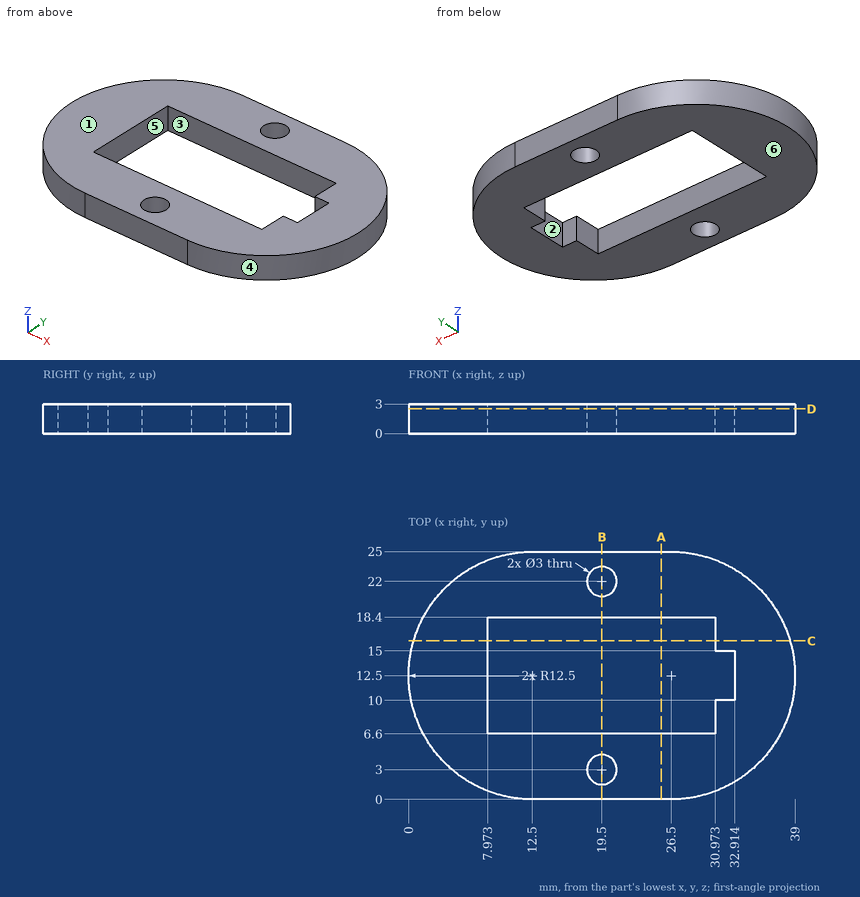
Drawing for the job (mm, zero at the part's lowest x, y, z). A direction names the side the tool comes from. Round coordinates to 2 decimals unless told otherwise and drop trailing zeros. Write each loop counter-clockwise with the first axis right and the second up, starting at its lowest first coordinate (ties: lowest second). Pieces come first, ordered by that corner, then holes. Notation, with made-up numbers: M -17,-38.5 L 1,-38.5 A14 cw 1,-24.5 Z; hole C -33,62 d4. An arc over 180 degrees is marked long. Answer in a Markdown table with one row per item.
1. Saw through at A-A (x = 25.5). List the corners of the cut face in (y, z).
Geometry check:
| item | result |
|---|---|
| outline | M 0,0 L 6.6,0 L 6.6,3 L 0,3 Z; M 18.4,0 L 25,0 L 25,3 L 18.4,3 Z |
2. Saw through at B-B (x = 19.5). List the corners of the cut face in (y, z), and give its area (3 significant figures).
Geometry check:
| item | result |
|---|---|
| outline | M 0,0 L 1.5,0 L 1.5,3 L 0,3 Z; M 4.5,0 L 6.6,0 L 6.6,3 L 4.5,3 Z; M 18.4,0 L 20.5,0 L 20.5,3 L 18.4,3 Z; M 23.5,0 L 25,0 L 25,3 L 23.5,3 Z |
| area | 21.6 mm2 |
3. Saw through at D-D (z = 2.5). List the corners of the cut face in (x, y).
Geometry check:
| item | result |
|---|---|
| outline | M 12.5,0 L 26.5,0 A12.5 ccw 26.5,25 L 12.5,25 A12.5 ccw Z; hole M 7.97,6.6 L 30.97,6.6 L 30.97,10 L 32.91,10 L 32.91,15 L 30.97,15 L 30.97,18.4 L 7.97,18.4 Z; hole C 19.5,3 d3; hole C 19.5,22 d3 |
4. Which spindle directions (+Z, -Z, +X, -X, +Y, -Y) get a long thin tool onto all of the face, cutting with end or side? Do the marked faces 5 and 6. Say none if no direction does.
Geometry check:
| item | result |
|---|---|
| face 5 | +Z, -Z |
| face 6 | -Z, +X, -X, +Y, -Y |
5. Saw through at C-C (y = 16). List the corners of the cut face in (x, z), and give its area (3 significant figures).
Geometry check:
| item | result |
|---|---|
| outline | M 0.5,0 L 7.97,0 L 7.97,3 L 0.5,3 Z; M 30.97,0 L 38.5,0 L 38.5,3 L 30.97,3 Z |
| area | 45.0 mm2 |
6. Probe L1, parallel to Y at x = 19.5, z = 2.3; L2, parallel to Y at x = 25, z = 0.35; L3, parallel to X at y = 12.5, z = 1.45. List the from-to ranges inside material, lowest first. Write a range as [from, to].
Geometry check:
| item | result |
|---|---|
| L1 | [0, 1.5], [4.5, 6.6], [18.4, 20.5], [23.5, 25] |
| L2 | [0, 6.6], [18.4, 25] |
| L3 | [0, 7.97], [32.91, 39] |
7. Mould opens along X. For the marked faces 1, 2, 3 and 4 say: +X half, -X half, draft (parallel to the pull), parting line (faces both ways), or undercut.
Geometry check:
| item | result |
|---|---|
| face 1 | draft |
| face 2 | undercut |
| face 3 | undercut |
| face 4 | +X half |
8. Flat gauge pins, fed straight in: P1, Ø0.9, axis at y = 14, z = 2, coming from the +X side; P2, Ø3, axis at x = 22, y = 16.5, coming from the +Z side; P3, Ø4, axis at x = 19.5, y = 22, coming from the -Z side; P4, Ø0.9, axis at y = 8.5, z = 1.5, coming from the -X side (1 decimal). Where does each tip first touch, or does it go through?
Geometry check:
| item | result |
|---|---|
| P1 | x = 38.96 |
| P2 | through |
| P3 | z = 0 |
| P4 | x = 0.5 |
